Read the model definition and answer for the solid it produces. Units are mm, in the model's axes. A direction names the side the tool comes from. Round coordinates to 2 decimals unless told otherwise and drop trailing zeros. Loops run counter-clockwise (first coordinate to the right, second up) from the corner with the lowest first, then second, coordinate; pieces in that order, holes last. Notation, with made-up numbers: (35.5, -37) - (53.5, -37) arc R23 cw to (53.5, -21) - close; hole circle Ø8 at (27.5, -12.5). An arc over 180 degrees is marked (long way). Use CSV: the item, a comma, the result in double quotes. Start each with the question number.
1. Consider line 1 along X through (y, z) = (-29, -25); line 2 along X through (y, z) = (14, 6.5); line 3 along Y through (x, z) = (11, -14). Determine where each line is inside the solid, lowest interval first.
2. Find section A-A (z = -25). Give the vertices of the cut face in (x, y), and give its area (3 significant figures).
3. Find section C-C (y = -11). Give the vertices of the cut face in (x, z).
4. Find section B-B (x = -7). Give the vertices of the cut face in (y, z), and give its area (3 significant figures).
5. A tool of negligible diameter and unlimited length cuts with its end or side. For faces 4 (the flat face through (0, -30.082, -10)), 5 (the flat face through (15, -25.082, -3)), 6 (the cylindrical face through (14.511, -17.667, 7.465)), from which of +Z, -Z, +X, -X, +Y, -Y can it reach the whole face along a straight path? Write none if from no direction.
6. Given pin 1 Ø10 at (x, y) = (-1, 3) entering from -Z; pin 2 Ø8 at (x, y) = (15.26, -15.28) entering from -Z; pin 3 Ø4 at (x, z) = (-14.94, -25) entering from +Y; pin 4 Ø2.5 at (x, y) = (16, -16) entering from +Z, each flat-ended and moving along its own axis, determine where each tip first touches the part or whether it passes through.
7. Determine the mould class of faces 1 (the flat face through (0, 19.918, 5)), 2 (the cylindrical face through (11.984, -3.837, 4.93)), 3 (the flat face through (-18.46, -25.52, -28.48)) for opening direction X: +X half, -X half, draft (parallel to the pull), parting line (faces both ways), or undercut.
8. Find section D-D (z = 4). Give the vertices of the cut face in (x, y), and give its area (3 significant figures).
Autodesk Inventor part; units mm, degrees
ref_plane "YZ Plane" through (0, 0, 0) normal (1, 0, 0) x (0, 1, 0)
ref_plane "XZ Plane" through (0, 0, 0) normal (0, 1, 0) x (-1, 0, 0)
ref_plane "XY Plane" through (0, 0, 0) normal (0, 0, 1) x (1, 0, 0)
sketch "Sketch1" plane through (0, 0, 0) normal (0, 0, 1) x (1, 0, 0)
  line L0 (20.0617, 19.9177) -> (20.0617, -20.0823)
  line L1 (20.0617, -20.0823) -> (-19.9383, -20.0823)
  line L2 (-19.9383, -20.0823) -> (-19.9383, 19.9177)
  line L3 (20.0617, 19.9177) -> (-19.9383, 19.9177)
  line L4 (-19.9383, 29.9177) -> (-19.9383, -30.0823)
  line L5 (15.2617, 19.9177) -> (15.2617, 15.1177)
  line L6 (15.2617, 19.9177) -> (20.0617, 19.9177) construction
  circle A0 centre (15.2617, 15.1177) radius 1.6
  line L7 (-19.9383, -0.0823) -> (20.0617, -0.0823)
  line L8 (0.0617, -20.0823) -> (0.0617, 19.9177)
  circle A1 centre (15.2617, -15.2823) radius 1.6
  circle A2 centre (-15.1383, -15.2823) radius 1.6
  circle A3 centre (-15.1383, 15.1177) radius 1.6
  arc A4 (10.0617, 7.4177) -> (10.0617, -7.5823) centre (0.0617, -0.0823) ccw
  line L9 (-12.4383, -0.0823) -> (2.0617, -0.0823)
  circle A5 centre (0.0617, -0.0823) radius 12.5
  point P0 (0, 0)
  dimension "d0" = 40
  dimension "d1" = 40
  dimension "d2" = 4.8
  dimension "d3" = 90
  dimension "d4" = 4.8
  dimension "d5" = 3.2
  dimension "d6" = 25
  dimension "d7" = 20
  dimension "d8" = 4.8
  dimension "d9" = 3.2
  dimension "d10" = 25
  dimension "d11" = 40
  dimension "d12" = 40
extrude "Extrusion1" add sketch "Sketch1" along normal blind 10 contours L0 L7 A5 A4 L8 L3 | L0 L1 L8 A4 A5 L7 | L8 A4 L7 L2 L3 | L1 L2 L7 A4 L8
sketch "Sketch2" plane through (-19.9383, -20.0823, 0) normal (0, -1, 0) x (1, 0, 0)
  line L0 (40, 0) -> (40, 10)
  line L1 (40, 10) -> (0, 10)
  line L2 (0, 10) -> (0, -30)
  line L3 (0, -30) -> (40, -30)
  line L4 (40, -30) -> (40, 10)
  point P0 (19.9383, 0)
  dimension "d15" = 40
  dimension "d21" = 40
extrude "Extrusion2" add sketch "Sketch2" along normal blind 10
chamfer "Chamfer1" distance 3 angle 45 2 edges at (-19.9383, 19.9177, 5) (20.0617, 19.9177, 5)
sketch "Sketch3" plane through (-19.9383, -20.0823, 0) normal (0, 1, 0) x (1, 0, 0)
  line L0 (0, 0) -> (0, 30)
  line L1 (0, 0) -> (5, 0)
  line L2 (5, 0) -> (5, 5)
  line L3 (5, 5) -> (0, 5)
  line L4 (0, 5) -> (0, 0)
  circle A0 centre (5, 5) radius 1.6
  line L5 (19.9383, 0) -> (19.9383, 30)
  line L6 (0, 15) -> (41.8735, 15)
  circle A1 centre (5, 25) radius 1.6
  circle A2 centre (34.8766, 5) radius 1.6
  circle A3 centre (34.8766, 25) radius 1.6
  dimension "d22" = 5
  dimension "d23" = 5
  dimension "d24" = 3.2
hole "Hole1" at (-14.9383, -20.0823, -25) at (14.9383, -20.0823, -25) at (14.9383, -20.0823, -5) at (-14.9383, -20.0823, -5) direction (0, -1, 0) diameter 3.2 end through all counterbore diameter 5 counterbore depth 5
sketch "Sketch4" plane through (0, 0, 10) normal (0, 0, 1) x (1, 0, 0)
  circle A0 centre (-15.1383, 15.1177) radius 1.6
  line L0 (0, 0) -> (-15.1383, 0)
  line L1 (-15.1383, 0) -> (-15.1383, 15.1177)
  line L2 (-15.1383, 15.1177) -> (0, 15.1177)
  line L3 (0, 15.1177) -> (0, 0)
  circle A1 centre (15.2617, -15.2823) radius 1.6
  line L4 (-15.1383, 15.1177) -> (15.2617, 15.1177)
  line L5 (15.2617, 15.1177) -> (15.2617, -15.2823)
  line L6 (15.2617, -15.2823) -> (-15.1383, -15.2823)
  line L7 (-15.1383, -15.2823) -> (-15.1383, 15.1177)
  circle A2 centre (-15.1383, 15.1177) radius 1.6
  circle A3 centre (15.2617, 15.1177) radius 1.6
  circle A4 centre (15.2617, 15.1177) radius 1.6
  circle A5 centre (15.2617, -15.2823) radius 1.6
  circle A6 centre (-15.1383, -15.2823) radius 1.6
hole "Hole2" at (-15.1383, 15.1177, 10) at (15.2617, 15.1177, 10) at (15.2617, -15.2823, 10) at (-15.1383, -15.2823, 10) direction (0, 0, -1) diameter 3.2 end through all counterbore diameter 5 counterbore depth 5
sketch "Sketch5" plane through (-19.9383, -30.0823, 0) normal (0, -1, 0) x (1, 0, 0)
  circle A0 centre (5, -25) radius 1.6
  circle A1 centre (34.8766, -25) radius 1.6
  circle A2 centre (34.8766, -5) radius 1.6
  point P0 (19.9383, 0)
  dimension "d39" = 26.6766
  dimension "d40" = 29.8766
  dimension "d41" = 20
sketch "Sketch6" plane through (-19.9383, -20.0823, 0) normal (0, 1, 0) x (1, 0, 0)
  line L0 (0, 0) -> (40, 0)
  line L1 (0, 30) -> (40, 30)
  line L2 (0, 0) -> (40, 0)
  line L3 (40, 0) -> (40, 30)
  line L4 (40, 30) -> (0, 30)
  line L5 (0, 30) -> (0, 0)
  point P0 (19.9383, 0)
extrude "Extrusion3" cut sketch "Sketch6" against normal blind 1
chamfer "Chamfer2" distance 3 angle 45 2 edges at (20.0617, -25.5823, -30) (-19.9383, -25.5823, -30)
properties part number "MotorMount"
Filled sheet:
1,line 1,"x = -19.94 to -16.54, -13.34 to 13.34, 16.54 to 20.06"
1,line 2,"x = -19.94 to -17.37, -12.9 to 13.03, 17.5 to 20.06"
1,line 3,"y = -30.08 to -21.08"
2,outline,"(-19.94, -30.08) - (-16.54, -30.08) - (-16.54, -25.08) - (-17.44, -25.08) - (-17.44, -21.08) - (-19.94, -21.08) - close; (-13.34, -30.08) - (13.34, -30.08) - (13.34, -25.08) - (12.44, -25.08) - (12.44, -21.08) - (-12.44, -21.08) - (-12.44, -25.08) - (-13.34, -25.08) - close; (16.54, -30.08) - (20.06, -30.08) - (20.06, -21.08) - (17.44, -21.08) - (17.44, -25.08) - (16.54, -25.08) - close"
2,area,"288 mm²"
3,outline,"(-19.94, 0) - (-6.03, 0) - (-6.03, 10) - (-19.94, 10) - close; (6.15, 0) - (20.06, 0) - (20.06, 10) - (6.15, 10) - close"
4,outline,"(-30.08, -30) - (-21.08, -30) - (-21.08, 0) - (-10.4, 0) - (-10.4, 10) - (-30.08, 10) - close; (10.23, 0) - (19.92, 0) - (19.92, 10) - (10.23, 10) - close"
4,area,"564 mm²"
5,face 4,"+Z, -Z, +X, -X, -Y"
5,face 5,"+Y"
5,face 6,"+Z"
6,pin 1,"passes through"
6,pin 2,"stops at z = 0"
6,pin 3,"stops at y = -25.08"
6,pin 4,"stops at z = 5"
7,face 1,"draft"
7,face 2,"undercut"
7,face 3,"-X half"
8,outline,"(-19.94, -30.08) - (20.06, -30.08) - (20.06, 16.92) - (17.06, 19.92) - (-16.94, 19.92) - (-19.94, 16.92) - close; hole circle Ø3.2 at (-15.14, -15.28); hole circle Ø3.2 at (-15.14, 15.12); hole circle Ø25 at (0.06, -0.08); hole circle Ø3.2 at (15.26, -15.28); hole circle Ø3.2 at (15.26, 15.12)"
8,area,"1,470 mm²"
